Here's the drawing with two shaded views (mm, measured from the low corner). I have some questions. A direction names the side the tool comes from. Round coordinates to 2 decimals unless told otherwise and drop trailing zeros. Loops run counter-clockwise (first coordinate to the right, second up) from the corner with the lowest first, then second, coordinate; pieces in that order, holes last. Notation, with made-up numbers: (12, 71.25) -> (48, 71.25) arc R15 cw to (48, 84.25) -> close; hole circle Ø5 at (23, 9). An arc over 180 degrees is marked (long way). One line per item, written item: value. Start each with the question number.
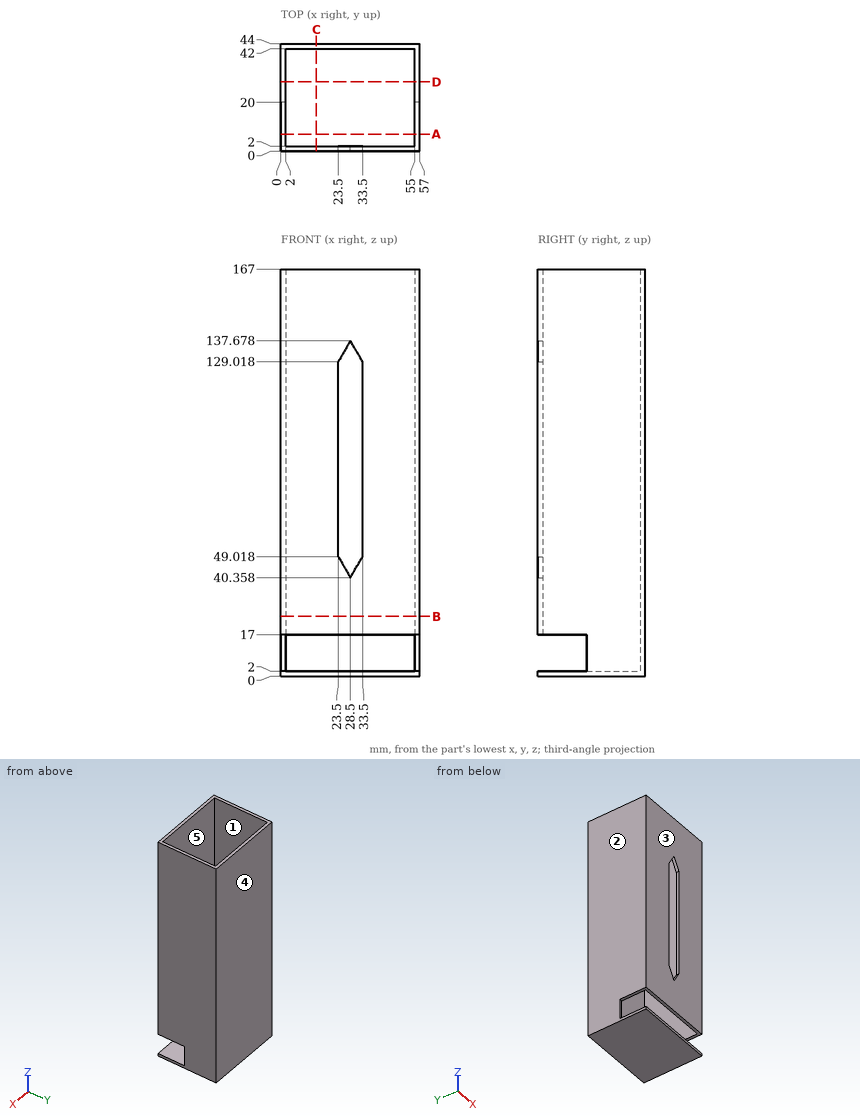
Q1. I want a section at C-C on x = 14.5. Please give me the cut outline in (y, z).
Q2. Which directions (+Z, -Z, +X, -X, +Y, -Y) give clear straight access to the entire face, cutting with the end or side of a thin tool? Please do the marked faces 1 and 2.
Q3. If we mould it in two halves opening along Y, with no side actions, what happens to the marked faces 3, 4 and 5? For each: released by +Y, released by -Y, zero draft, split by the parting line, or undercut.
Q4. I want a section at A-A on y = 7. Please give me the cut outline in (x, z).
Q5. Will these pins go through, and if not, where does the flat tip stop? P1, Ø2, axis at x = 55.5, z = 12.5, coming from the -Y side; P2, Ø1, axis at x = 17, y = 23.5, coming from the +Z side.
Q6. If I drill on line 1 along X through (y, z) = (23, 96); line 2 along Y through (x, z) = (35, 35); line 3 along Z through (x, y) = (26, 6.5), over which ranges is the centre line in solid material (lowest first)?
Q7. I want a section at D-D on y = 28.5. Please give me the cut outline in (x, z).
Q8. I want a section at B-B on z = 24.5. Please give me the cut outline in (x, y), plus the area to 3 significant figures.
Answers below:
1. outline: (0, 0) -> (44, 0) -> (44, 167) -> (42, 167) -> (42, 2) -> (0, 2) -> close; (0, 17) -> (2, 17) -> (2, 167) -> (0, 167) -> close
2. face 1: +Z
2. face 2: +Z, -Z, -X, +Y, -Y
3. face 3: released by -Y
3. face 4: released by +Y
3. face 5: undercut
4. outline: (0, 0) -> (57, 0) -> (57, 2) -> (0, 2) -> close; (0, 17) -> (2, 17) -> (2, 167) -> (0, 167) -> close; (55, 17) -> (57, 17) -> (57, 167) -> (55, 167) -> close
5. P1: stops at y = 20
5. P2: stops at z = 2
6. line 1: x = 0 to 2, 55 to 57
6. line 2: y = 0 to 2, 42 to 44
6. line 3: z = 0 to 2
7. outline: (0, 0) -> (57, 0) -> (57, 167) -> (55, 167) -> (55, 2) -> (2, 2) -> (2, 167) -> (0, 167) -> close
8. outline: (0, 0) -> (57, 0) -> (57, 44) -> (0, 44) -> close; hole (2, 2) -> (55, 2) -> (55, 42) -> (2, 42) -> close
8. area: 388 mm^2
